For this review, take the finished solid that the model builds, in its own axes (mm). A direction names the side the tool comes from. Round coordinates to 2 decimals unless told otherwise and drop trailing zeros. Order: outer loops, then holes, each group sorted by start corner. A loop starts at its lowest first (then second) coordinate and runs counter-clockwise, first axis right, second up. Notation, with made-up numbers: M -26.5,37.5 L -18.5,37.5 A18 cw -18.5,45.5 Z; hole C -38,55 d5. An arc over 180 degrees is marked long. Answer as a JSON object with one key per item and string values.
from build123d import *

# Parameters (mm, degrees)
PAD002_DEPTH  = 60
SKETCH005_R   = 90
SKETCH005_R_2 = 53
PAD004_DEPTH  = 100
PAD003_DEPTH  = 60
SKETCH007_R   = 53
PAD006_DEPTH  = 140
PAD005_DEPTH  = 60
PAD_DEPTH     = 10


with BuildPart() as body002:
    # Sketch003 → Pad002 (new body)
    with BuildSketch(Plane.XZ):
        Polygon((0, 108), (-23, 101.837169), (-23, 68.162831), (0, 62), (23, 68.162831), (23, 101.837169), align=None)
    extrude(amount=PAD002_DEPTH)


with BuildPart() as body:
    # Sketch → Revolution (revolve)
    with BuildSketch(Plane.XZ):
        Polygon((47, 135), (47, 0), (53, 0), (53, 142), (51, 142), (51, 150), (49, 150), (49, 135), align=None)
    revolve(axis=Axis((0, 0, 0), (0, 0, 1)))


with BuildPart() as body004:
    # Sketch005 → Pad004 (new body)
    with BuildSketch(Plane.XY):
        Circle(SKETCH005_R)
        Circle(SKETCH005_R_2, mode=Mode.SUBTRACT)
    extrude(amount=PAD004_DEPTH)


with BuildPart() as fusion:
    # Sketch004 → Pad003 (new body, symmetric)
    with BuildSketch(Plane.XZ):
        Polygon((0, 62), (-57.95555, 77.529143), (-57.95555, 0), (0, 0), (57.95555, 0), (57.95555, 77.529143), align=None)
    extrude(amount=PAD003_DEPTH, both=True)

    # Cut: cut Body004
    add(body004.part, mode=Mode.SUBTRACT)

    # Fusion: union Body
    add(body.part)


with BuildPart() as body006:
    # Sketch007 → Pad006 (new body)
    with BuildSketch(Plane.XY):
        Circle(SKETCH007_R)
    extrude(amount=PAD006_DEPTH)


with BuildPart() as cut002:
    # Sketch006 → Pad005 (new body)
    with BuildSketch(Plane.XZ):
        Polygon((0, 110), (-25, 103.30127), (-25, 66.69873), (0, 60), (25, 66.69873), (25, 103.30127), align=None)
    extrude(amount=PAD005_DEPTH)

    # Cut001: cut Body006
    add(body006.part, mode=Mode.SUBTRACT)

    # Fusion001: union Fusion
    add(fusion.part)

    # Cut002: cut Body002
    add(body002.part, mode=Mode.SUBTRACT)


with BuildPart() as body007:
    # Body007 base: copy of Cut002
    add(cut002.part)

    # Sketch008 → Pad (new body)
    with BuildSketch(Plane.XY):
        Polygon((77.38084, -39.037455), (72.5, -50), (-72.5, -50), (-77.38084, -39.037455), (-50, 0), (-58.436557, 49.283106), (-49.470337, 57.258499), (0, 50), (49.470337, 57.258499), (58.436557, 49.283106), (50, 0), align=None)
    extrude(amount=PAD_DEPTH)


with BuildPart() as fusion002:
    # Fusion002 base: copy of Cut002
    add(cut002.part)

    # Fusion002: union Body007
    add(body007.part)


solid = fusion002.part
1) Add section C-C on y = -8. State the section outline as (x, z) points, and give its area (3 significant figures).
Geometry check:
{"outline": "M -55.61,0 L 55.61,0 L 55.61,10 L 52.39,10 L 52.39,142 L 50.37,142 L 50.37,150 L 48.34,150 L 48.34,135 L 46.31,135 L 46.31,74.41 L 0,62 L -46.31,74.41 L -46.31,135 L -48.34,135 L -48.34,150 L -50.37,150 L -50.37,142 L -52.39,142 L -52.39,10 L -55.61,10 Z", "area": "8,110 mm²"}
2) Mouldability with a two-part tool opening along X and no side actions: class faces 4 (the flat face through (-45, -50, 5)), 5 (the flat face through (-15.45, -54.75, 64.14)), 6 (the flat face through (30.288, 54.444, 4.93)) as +X half, -X half, draft (parallel to the pull), parting line (faces both ways), or undercut.
Geometry check:
{"face 4": "draft", "face 5": "-X half", "face 6": "undercut"}
3) Add section A-A on x = 5. State the section outline as (y, z) points.
Geometry check:
{"outline": "M -60,61.34 L -52.76,61.34 L -52.76,0 L 52.76,0 L 52.76,142 L 50.75,142 L 50.75,150 L 48.74,150 L 48.74,135 L 46.73,135 L 46.73,63.34 L -60,63.34 Z; M -60,106.66 L -46.73,106.66 L -46.73,135 L -48.74,135 L -48.74,150 L -50.75,150 L -50.75,142 L -52.76,142 L -52.76,108.66 L -60,108.66 Z"}
4) Insertion check: P1, Ø3, axis at x = -38.5, y = 10.5, coming from the +Z side; P2, Ø12, axis at y = 12.5, z = 90, coming from the -X side; P3, Ø6, axis at x = -11, z = 30.5, coming from the -Y side. Each pin has a flat end and moves straight along its axis. Give the tip position at first contact, or say it passes through.
Geometry check:
{"P1": "stops at z = 72.72", "P2": "stops at x = -52.6", "P3": "stops at y = -52.39"}
5) Machinability: for faces 1 (the cylindrical face through (-11.056, -49.787, 146.056)), 2 (the flat face through (-65.284, -21.791, 4.93)), 3 (the flat face through (25, -53, 85)), which of the approach directions +Z, -Z, +X, -X, +Y, -Y give a long, thin tool a straight path to every point of the face, cutting with its end or side? Answer none if there is none.
Geometry check:
{"face 1": "+Z", "face 2": "+Z, -Z, -X", "face 3": "+Z, +X, -Y"}
6) Add section D-D on x = -27. State the section outline as (y, z) points.
Geometry check:
{"outline": "M -50,0 L 53.96,0 L 53.96,10 L 45.61,10 L 45.61,142 L 43.27,142 L 43.27,150 L 40.89,150 L 40.89,135 L 38.47,135 L 38.47,69.23 L -38.47,69.23 L -38.47,135 L -40.89,135 L -40.89,150 L -43.27,150 L -43.27,142 L -45.61,142 L -45.61,10 L -50,10 Z"}
7) For L1, parallel to Y at x = 0, z = 141; L2, parallel to Y at x = 0, z = 145; L3, parallel to X at y = 0, z = 106, list the stretches that pass through material, from the lowest coordinate up.
Geometry check:
{"L1": "y = -53 to -49, 49 to 53", "L2": "y = -51 to -49, 49 to 51", "L3": "x = -53 to -47, 47 to 53"}
8) Add section B-B on z = 140. State the section outline as (x, y) points.
Geometry check:
{"outline": "C 0,0 d106; hole C 0,0 d98"}
